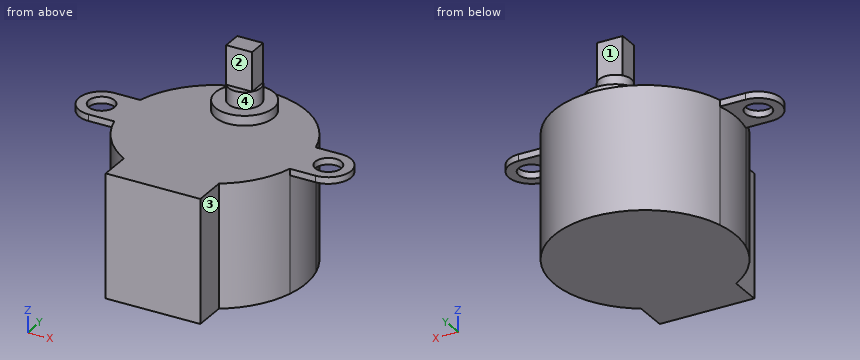
from build123d import *

# Parameters (mm, degrees)
ESBO_O2_R                = 14
RESSALTO_EXTRUS_O2_DEPTH = 19
ESBO_O3_W                = 14.6
ESBO_O3_H                = 5
RESSALTO_EXTRUS_O3_DEPTH = 19
ESBO_O4_W                = 10
ESBO_O4_H                = 7
RESSALTO_EXTRUS_O4_DEPTH = 19
RESSALTO_EXTRUS_O5_DEPTH = 19
ESBO_O6_R                = 2
CORTE_EXTRUS_O1_DEPTH    = 35.551542095
CORTE_EXTRUS_O2_DEPTH    = 35.551542095
CORTE_EXTRUS_O3_DEPTH    = 35.551542095
ESBO_O9_R                = 4.5
RESSALTO_EXTRUS_O7_DEPTH = 20.5
ESBO_O10_R               = 2.5
RESSALTO_EXTRUS_O8_DEPTH = 2.5
ESBO_O11_W               = 4
ESBO_O11_H               = 3
RESSALTO_EXTRUS_O9_DEPTH = 29
CORTE_EXTRUS_O4_DEPTH    = 18
CORTE_EXTRUS_O5_DEPTH    = 18


with BuildPart() as part:
    # Esboço2 → Ressalto-extrusão2 (new body)
    with BuildSketch(Plane.XY):
        Circle(ESBO_O2_R)
    extrude(amount=RESSALTO_EXTRUS_O2_DEPTH)

    # Esboço3 → Ressalto-extrusão3 (add)
    with BuildSketch(Plane.XY.offset(19)):
        with Locations((0.104281732, -14.40160663)):
            Rectangle(ESBO_O3_W, ESBO_O3_H)
    extrude(amount=-RESSALTO_EXTRUS_O3_DEPTH)

    # Esboço4 → Ressalto-extrusão4 (add)
    with BuildSketch(Plane.XY.offset(19)):
        with Locations((18.39112555, 0)):
            Rectangle(ESBO_O4_W, ESBO_O4_H)
    extrude(amount=-RESSALTO_EXTRUS_O4_DEPTH)

    # Esboço5 → Ressalto-extrusão5 (add)
    with BuildSketch(Plane.XY.offset(19)):
        Polygon((-13.354036811, 3.5), (-23.354036811, 3.5), (-23.354036811, -3.5), (-13.354036811, -3.5), (-13.354036811, 0), align=None)
    extrude(amount=-RESSALTO_EXTRUS_O5_DEPTH)

    # Esboço6 → Corte-extrusão1 (cut, through all)
    with BuildSketch(Plane.XY.offset(19)):
        with Locations((-17.5, 0)):
            Circle(ESBO_O6_R)
        with Locations((17.5, 0)):
            Circle(ESBO_O6_R)
    extrude(amount=-CORTE_EXTRUS_O1_DEPTH, mode=Mode.SUBTRACT)

    # Esboço7 → Corte-extrusão2 (cut, through all)
    with BuildSketch(Plane.XY):
        with BuildLine():
            Line((-17.5, 3.5), (-23.354036811, 3.5))
            Line((-23.354036811, 3.5), (-23.354036811, -3.5))
            Line((-23.354036811, -3.5), (-17.5, -3.5))
            ThreePointArc((-17.5, -3.5), (-21, 0), (-17.5, 3.5))
        make_face()
    extrude(amount=CORTE_EXTRUS_O2_DEPTH, mode=Mode.SUBTRACT)

    # Esboço8 → Corte-extrusão3 (cut, through all)
    with BuildSketch(Plane.XY):
        with BuildLine():
            Line((17.5, 3.5), (23.39112555, 3.5))
            Line((23.39112555, 3.5), (23.39112555, -3.5))
            Line((23.39112555, -3.5), (17.5, -3.5))
            ThreePointArc((17.5, -3.5), (21, 0), (17.5, 3.5))
        make_face()
    extrude(amount=CORTE_EXTRUS_O3_DEPTH, mode=Mode.SUBTRACT)

    # Esboço9 → Ressalto-extrusão7 (add)
    with BuildSketch(Plane.XY):
        with Locations((0, 8)):
            Circle(ESBO_O9_R)
    extrude(amount=RESSALTO_EXTRUS_O7_DEPTH)

    # Esboço10 → Ressalto-extrusão8 (add)
    with BuildSketch(Plane.XY.offset(20.5)):
        with Locations((0, 8)):
            Circle(ESBO_O10_R)
    extrude(amount=RESSALTO_EXTRUS_O8_DEPTH)

    # Esboço11 → Ressalto-extrusão9 (add)
    with BuildSketch(Plane.XY):
        with Locations((0, 8)):
            Rectangle(ESBO_O11_W, ESBO_O11_H)
    extrude(amount=RESSALTO_EXTRUS_O9_DEPTH)

    # Esboço12 → Corte-extrusão4 (cut)
    with BuildSketch(Plane(origin=(0, 0, 0), x_dir=(-1, 0, 0), z_dir=(0, 0, -1))):
        with BuildLine():
            Line((-17.5, -3.5), (-13.555441712, -3.5))
            ThreePointArc((-13.555441712, -3.5), (-14, 0), (-13.555441712, 3.5))
            Line((-13.555441712, 3.5), (-17.5, 3.5))
            ThreePointArc((-17.5, 3.5), (-21, 0), (-17.5, -3.5))
        make_face()
    extrude(amount=-CORTE_EXTRUS_O4_DEPTH, mode=Mode.SUBTRACT)

    # Esboço13 → Corte-extrusão5 (cut)
    with BuildSketch(Plane(origin=(0, 0, 0), x_dir=(-1, 0, 0), z_dir=(0, 0, -1))):
        with BuildLine():
            Line((13.555441712, -3.5), (17.5, -3.5))
            ThreePointArc((17.5, -3.5), (21, 0), (17.5, 3.5))
            Line((17.5, 3.5), (13.555441712, 3.5))
            ThreePointArc((13.555441712, 3.5), (14, 0), (13.555441712, -3.5))
        make_face()
    extrude(amount=-CORTE_EXTRUS_O5_DEPTH, mode=Mode.SUBTRACT)


solid = part.part
The listing builds one solid part. Answer for the finished solid, in the listing's coordinates (mm). Face numbers are marked on the shaded views. A direction names the side the tool comes from. Round coordinates to 2 decimals unless told otherwise and drop trailing zeros. Write each loop counter-clockwise with the first axis right and the second up, starting at its lowest first coordinate (ties: lowest second). Pieces come first, ordered by that corner, then holes. Notation, with made-up numbers: M 61,84.25 L 73,84.25 A18 cw 73,90.25 Z; hole C 85.5,87.5 d8. An arc over 180 degrees is marked long. Write each question's results on one line, items separated by ' | '. Start each with the question number.
Item 1: Straight lines are drawn through the part: probe 1 along Y at (x, z) = (17.5, 18.75); probe 2 along Z at (x, y) = (18.5, 3); probe 3 along Z at (x, y) = (1, -8). For each, find the intervals that lie inside material, in ascending order.
Item 2: Find section D-D on x = 0. Write down the section's boundary in (y, z).
Item 3: Find section B-B on x = -16. Write down the section's boundary in (y, z), and give its area (3 significant figures).
Item 4: Find section A-A on y = 0. Write down the section's boundary in (x, z), and give its area (3 significant figures).
Item 5: Given pin 1 Ø3 at (x, y) = (8, 1) entering from +Z; pin 2 Ø8 at (y, z) = (8, 14) entering from -X; pin 3 Ø12 at (y, z) = (-13.5, 23.5) entering from +X; pin 4 Ø1.1 at (x, y) = (1, 10) entering from +Z, each flat-ended and moving along its own axis, determine where each tip first touches the part or whether it passes through.
Item 6: Which of the six approach directions +Z, -Z, +X, -X, +Y, -Y give full straight-line access (tool end or side, diameter ignored) to the marked faces 1, 2, 3 and 4?
Answer block:
1) probe 1: y = -3.5 to -2, 2 to 3.5 | probe 2: z = 18 to 19 | probe 3: z = 0 to 19
2) outline: M -16.9,0 L 14,0 L 14,19 L 12.5,19 L 12.5,20.5 L 10.5,20.5 L 10.5,23 L 9.5,23 L 9.5,29 L 6.5,29 L 6.5,23 L 5.5,23 L 5.5,20.5 L 3.5,20.5 L 3.5,19 L -16.9,19 Z
3) outline: M -3.5,18 L -1.32,18 L -1.32,19 L -3.5,19 Z; M 1.32,18 L 3.5,18 L 3.5,19 L 1.32,19 Z | area: 4.35 mm²
4) outline: M -21,18 L -19.5,18 L -19.5,19 L -21,19 Z; M -15.5,18 L -14,18 L -14,0 L 14,0 L 14,18 L 15.5,18 L 15.5,19 L -15.5,19 Z; M 19.5,18 L 21,18 L 21,19 L 19.5,19 Z | area: 538 mm²
5) pin 1: stops at z = 19 | pin 2: stops at x = -13.42 | pin 3: stops at x = 10.25 | pin 4: stops at z = 29
6) face 1: +Z, +X, -X, +Y | face 2: +Z, +X, -X, -Y | face 3: +Z, -Z, +X, -Y | face 4: +Z
